CAD build for the part. Positions are in the model's coordinates, mm. A direction names the side the tool comes from. Give positions to 0.01 mm unless a question says otherwise; leave off trailing zeros. Order: outer loops, then holes, each group sorted by start corner. A loop starts at its lowest first (then second) coordinate and runs counter-clockwise, first axis right, second up.
Item 1: Band-saw the part on C-C on x = -56.5. Give the cut face in (y, z), plus the area to 3 significant figures.
Item 2: Two-plate mould, pull along Z, no slides. Class faces 4 (the flat face through (108.944, 17.595, -102.517)), 5 (the flat face through (-45.91, -17.43, 4.06)), 6 (the cylindrical face through (109, 0, -156)): released by +Z, released by -Z, zero draft, split by the parting line, or undercut.
Item 3: Flat gauge pins, fed straight in: P1, Ø4, axis at x = 37.5, z = -106, coming from the +Y side; P2, Ø3, axis at y = 5.5, z = -16, coming from the -X side; P3, Ø25, axis at y = -9, z = -149, coming from the -X side. Where does each tip first touch, or does it go through?
Item 4: Band-saw the part on D-D on x = 94.5. Give the cut face in (y, z).
Item 5: Wall check: L1, parallel to Z at x = 93.5, y = 0; L2, parallel to Z at x = 4, y = -16; L3, parallel to X at y = 6, z = -90.5. Give the ranges that are in metal, low to high.
Item 6: Which spindle directions (+Z, -Z, +X, -X, +Y, -Y) get a long thin tool onto all of the face, cutting with end or side? Do faces 1 (the flat face through (105, 0.4, -104.7)), 2 (the flat face through (2.483, -17.595, 4.056)), 3 (the cylindrical face through (18.58, -2.11, 4.06)). Say none if no direction does.
Item 7: Band-saw the part on A-A on z = -161.5. Give the cut face in (x, y), plus the area to 3 significant figures.
Item 8: Band-saw the part on B-B on y = 15. Give the cut face in (x, z), plus the area to 3 significant figures.
```python
from build123d import *

# Parameters (mm, degrees)
SWEEP3_PROFILE_R     = 21.5
CUT_SWEEP1_PROFILE_R = 20
SKETCH23_R           = 5.5
SKETCH23_R_2         = 21.5
SKETCH23_R_3         = 20
BOSS_EXTRUDE2_DEPTH  = 8
BOSS_EXTRUDE3_START  = 8
SKETCH26_R           = 5.5
SKETCH26_R_2         = 21.5
SKETCH26_R_3         = 20
BOSS_EXTRUDE3_DEPTH  = 8


with BuildPart() as part:
    # Sweep3: sweep along a path in Sketch1
    with BuildLine(Plane(origin=(0, 0, 0), x_dir=(1, 0, 0), z_dir=(0, 1, 0))) as sweep3_path:
        Line((105, 126.5), (43.5, 126.5))
        ThreePointArc((43.5, 126.5), (-2.461940777, 107.461940777), (-21.5, 61.5))
        Line((-21.5, 61.5), (-21.5, 0))
    # Sweep3 profile (on start of the path) → Sweep3 (sweep)
    with BuildSketch(Plane(origin=(105, 0, -126.5), x_dir=(0, 0, -1), z_dir=(-1, 0, 0))):
        Circle(SWEEP3_PROFILE_R)
    sweep(path=sweep3_path.line)

    # Cut-Sweep1: sweep along a path in Sketch1_5
    with BuildLine(Plane(origin=(0, 0, 0), x_dir=(1, 0, 0), z_dir=(0, 1, 0))) as cut_sweep1_path:
        Line((105, 126.5), (43.5, 126.5))
        ThreePointArc((43.5, 126.5), (-2.461940777, 107.461940777), (-21.5, 61.5))
        Line((-21.5, 61.5), (-21.5, 0))
    # Cut-Sweep1 profile (on start of the path) → Cut-Sweep1 (sweep, cut)
    with BuildSketch(Plane(origin=(105, 0, -126.5), x_dir=(0, 0, -1), z_dir=(-1, 0, 0))):
        Circle(CUT_SWEEP1_PROFILE_R)
    sweep(path=cut_sweep1_path.line, mode=Mode.SUBTRACT)

    # Sketch23 → Boss-Extrude2 (add)
    # profile 1 of 2: a face of its own
    with BuildSketch(Plane(origin=(105, 0, 0), x_dir=(0, 0, -1), z_dir=(1, 0, 0))):
        with BuildLine():
            Line((165.964285714, 11.67562217), (135.428571429, 23.35124434))
            ThreePointArc((135.428571429, 23.35124434), (126.5, 25), (117.571428571, 23.35124434))
            Line((117.571428571, 23.35124434), (87.035714286, 11.67562217))
            ThreePointArc((87.035714286, 11.67562217), (79, 0), (87.035714286, -11.67562217))
            Line((87.035714286, -11.67562217), (117.571428571, -23.35124434))
            ThreePointArc((117.571428571, -23.35124434), (126.5, -25), (135.428571429, -23.35124434))
            Line((135.428571429, -23.35124434), (165.964285714, -11.67562217))
            ThreePointArc((165.964285714, -11.67562217), (174, 0), (165.964285714, 11.67562217))
        make_face()
        with Locations((161.5, 0)):
            Circle(SKETCH23_R, mode=Mode.SUBTRACT)
        with Locations((91.5, 0)):
            Circle(SKETCH23_R, mode=Mode.SUBTRACT)
        with Locations((126.5, 0)):
            Circle(SKETCH23_R_2, mode=Mode.SUBTRACT)
    # profile 2 of 2: a face of its own
    with BuildSketch(Plane(origin=(105, 0, 0), x_dir=(0, 0, -1), z_dir=(1, 0, 0))):
        with Locations((126.5, 0)):
            Circle(SKETCH23_R_2)
        with Locations((126.5, 0)):
            Circle(SKETCH23_R_3, mode=Mode.SUBTRACT)
    extrude(amount=BOSS_EXTRUDE2_DEPTH)

    # Sketch26 → Boss-Extrude3 (add)
    # profile 1 of 2: a face of its own
    with BuildSketch(Plane.XY.offset(BOSS_EXTRUDE3_START)):
        with BuildLine():
            Line((17.964285714, 11.67562217), (-12.571428571, 23.35124434))
            ThreePointArc((-12.571428571, 23.35124434), (-21.5, 25), (-30.428571429, 23.35124434))
            Line((-30.428571429, 23.35124434), (-60.964285714, 11.67562217))
            ThreePointArc((-60.964285714, 11.67562217), (-69, 0), (-60.964285714, -11.67562217))
            Line((-60.964285714, -11.67562217), (-30.428571429, -23.35124434))
            ThreePointArc((-30.428571429, -23.35124434), (-21.5, -25), (-12.571428571, -23.35124434))
            Line((-12.571428571, -23.35124434), (17.964285714, -11.67562217))
            ThreePointArc((17.964285714, -11.67562217), (26, 0), (17.964285714, 11.67562217))
        make_face()
        with Locations((13.5, 0)):
            Circle(SKETCH26_R, mode=Mode.SUBTRACT)
        with Locations((-56.5, 0)):
            Circle(SKETCH26_R, mode=Mode.SUBTRACT)
        with Locations(Location((-21.5, 0, 0), (0, 0, 180))):
            Circle(SKETCH26_R_2, mode=Mode.SUBTRACT)
    # profile 2 of 2: a face of its own
    with BuildSketch(Plane.XY.offset(BOSS_EXTRUDE3_START)):
        with Locations(Location((-21.5, 0, 0), (0, 0, 180))):
            Circle(SKETCH26_R_2)
        with Locations(Location((-21.5, 0, 0), (0, 0, 180))):
            Circle(SKETCH26_R_3, mode=Mode.SUBTRACT)
    extrude(amount=-BOSS_EXTRUDE3_DEPTH)


solid = part.part
```
The answers:
1. outline: (-13.38, 0) - (-5.5, 0) - (-5.5, 8) - (-13.38, 8) - close; (5.5, 0) - (13.38, 0) - (13.38, 8) - (5.5, 8) - close
1. area: 126 mm2
2. face 4: released by +Z
2. face 5: zero draft
2. face 6: undercut
3. P1: stops at y = 11.61
3. P2: stops at x = -42.62
3. P3: stops at x = 2.77
4. outline: circle Ø43 at (0, -126.5); hole circle Ø40 at (0, -126.5)
5. L1: z = -148 to -146.5, -106.5 to -105
5. L2: z = -130.33 to -127.6, -96.84 to -93.19, 0 to 8
5. L3: x = -37.09 to -35.42, 7.89 to 9.94, 105 to 113
6. face 1: none
6. face 2: +Z, +X, -Y
6. face 3: +Z
7. outline: (105, -13.38) - (113, -13.38) - (113, -5.5) - (105, -5.5) - close; (105, 5.5) - (113, 5.5) - (113, 13.38) - (105, 13.38) - close
7. area: 126 mm2
8. outline: (-52.27, 0) - (-36.9, 0) - (-36.9, -61.5) arc R80.4 ccw to (43.5, -141.9) - (105, -141.9) - (105, -157.27) - (113, -157.27) - (113, -139.73) - (43.5, -139.73) arc R78.23 cw to (-34.73, -61.5) - (-34.73, 8) - (-52.27, 8) - close; (-8.27, -61.5) arc R51.77 ccw to (43.5, -113.27) - (113, -113.27) - (113, -95.73) - (105, -95.73) - (105, -111.1) - (43.5, -111.1) arc R49.6 cw to (-6.1, -61.5) - (-6.1, 0) - (9.27, 0) - (9.27, 8) - (-8.27, 8) - close
8. area: 1,540 mm2
